Could you check a few things on this model? Use its own coordinates, in mm. A direction names the side the tool comes from. Coordinates: 2 decimals unless noted, no trailing zeros. Write each loop counter-clockwise with the first axis right and the second up, starting at its lowest first coordinate (ties: lowest second). Pieces come first, ordered by that corner, then holes.
Autodesk Inventor part; units mm, degrees
ref_plane "YZ Plane" through (0, 0, 0) normal (1, 0, 0) x (0, 1, 0)
ref_plane "XZ Plane" through (0, 0, 0) normal (0, 1, 0) x (-1, 0, 0)
ref_plane "XY Plane" through (0, 0, 0) normal (0, 0, 1) x (1, 0, 0)
sketch "Sketch1" plane through (0, 0, 0) normal (0, 1, 0) x (-1, 0, 0)
  circle A0 centre (0, 0) radius 4.7625
  dimension "d0" = 9.525
extrude "Extrusion1" add sketch "Sketch1" along normal blind 304.8
thread "Thread1"
sketch "Sketch2" plane through (0, 304.8, 0) normal (0, 1, 0) x (1, 0, 0)
  circle A0 centre (0, 0) radius 4.7625
  arc A1 (1.7227, -2.667) -> (-1.7227, -2.667) centre (0, 0) ccw
  line L0 (-1.7227, -2.667) -> (1.7227, -2.667)
  dimension "d5" = 6.35
  dimension "d6" = 2.667
extrude "Extrusion2" cut sketch "Sketch2" against normal blind 9.525
sketch "Sketch3" plane through (0, 0, 0) normal (0, -1, 0) x (1, 0, 0)
  circle A0 centre (0, 0) radius 4.7625
  circle A1 centre (0, 0) radius 3.175
  dimension "d9" = 6.35
extrude "Extrusion3" cut sketch "Sketch3" against normal blind 25.4
properties part number "acmeScrew"
Item 1: If I drill on line 1 along Y through (x, z) = (-0.25, -3.5) (3 decimals); line 2 along X through (y, z) = (225.5, 0.75); line 3 along Z through (x, y) = (-0.25, 12), over which ranges is the centre line in solid material (lowest first)?
Item 2: I want a section at C-C, the plane y = 99. List the corners of the cut face in (x, z) for me (1 decimal), then the cut area to 3 significant figures.
Item 3: Which directions (+Z, -Z, +X, -X, +Y, -Y) give clear straight access to the entire face, cutting with the end or side of a thin tool? Please do faces 1 (the cylindrical face through (3.78, 158.45, 2.9)), 2 (the cylindrical face through (-0.69, 12.52, -3.1)), 3 (the cylindrical face through (0.114, 300.104, -3.173)).
Item 4: I want a section at B-B, the plane x = 0. List the corners of the cut face in (y, z) for me (1 decimal), then the cut area to 3 significant figures.
Item 5: I want a section at A-A, the plane z = 0. List the corners of the cut face in (x, y) for me (1 decimal), then the cut area to 3 significant figures.
Item 6: Will these pins go through, and if not, where does the flat tip stop? pin 1 Ø3 at (x, y) = (2, 87) entering from -Z; pin 2 Ø4 at (x, y) = (-0.5, 301) entering from +Z; pin 3 Ø1.5 at (x, y) = (2.5, 227.5) entering from -Z.
Taken from the geometry:
1. line 1: y = 25.4 to 295.275
1. line 2: x = -4.7 to 4.7
1. line 3: z = -3.17 to 3.17
2. outline: circle Ø9.5 at (0, 0)
2. area: 71.3 mm2
3. face 1: +Y, -Y
3. face 2: -Y
3. face 3: +Y
4. outline: (0, -3.2) - (25.4, -3.2) - (25.4, -4.8) - (295.3, -4.8) - (295.3, -3.2) - (304.8, -3.2) - (304.8, 2.7) - (295.3, 2.7) - (295.3, 4.8) - (25.4, 4.8) - (25.4, 3.2) - (0, 3.2) - close
4. area: 2,790 mm2
5. outline: (-4.8, 25.4) - (-3.2, 25.4) - (-3.2, 0) - (3.2, 0) - (3.2, 25.4) - (4.8, 25.4) - (4.8, 295.3) - (3.2, 295.3) - (3.2, 304.8) - (-3.2, 304.8) - (-3.2, 295.3) - (-4.8, 295.3) - close
5. area: 2,790 mm2
6. pin 1: stops at z = -4.74
6. pin 2: stops at z = 2.67
6. pin 3: stops at z = -4.43
